Read the model definition and answer for the solid it produces. Units are mm, in the model's axes. A direction names the side the tool comes from. Round coordinates to 2 decimals unless told otherwise and drop trailing zeros. Order: outer loops, then holes, each group sorted by start corner. A loop starts at its lowest first (then second) coordinate and runs counter-clockwise, first axis right, second up. Notation, with made-up numbers: (-25, 89) -> (-5, 89) arc R11 cw to (-5, 101) -> close; hole circle Ø5 at (8, -18.75). An arc over 180 degrees is marked (long way). Use a Markdown table: item, result. Add a question column.
1. Section C-C, the plane z = 9.5 is taken. Give the vertices of the cut face in (x, y), then the cut area to 3 significant figures.
2. The mould has two halves that part along X. Classify faces 3 (the face through (-400, -200, -75)), 4 (the face through (419.524, -98.6, 70.664)), 5 (the face through (-419.524, -98.6, 79.336)): +X half, -X half, draft (parallel to the pull), parting line (faces both ways), or undercut.
3. Consider L1, parallel to Y at x = -26, z = 75.5; L2, parallel to X at y = -182, z = -71; L3, parallel to X at y = -56, z = 78.5. Determine where each line is inside the solid, lowest interval first. Write a range as [from, to].
4. Given pin 1 (3 mm diameter, centred on y = 56.5, z = 21, fed in from -X); pin 2 (8 mm diameter, centred on x = -234, z = -12, fed in from -Y), each flat-ended and moving along its own axis, determine where each tip first touches the part or whether it passes through.
5. Section D-D, the plane z = 75 is taken. Give the vertices of the cut face in (x, y), then the cut area to 3 significant figures.
6. Section A-A, the plane y = -19.5 is taken. Give the vertices of the cut face in (x, z), then the cut area to 3 significant figures.
7. Section B-B, the plane x = 400 is taken. Give the vertices of the cut face in (y, z).
8. For faces 1 (the face through (-380.476, -98.6, -79.336)), 2 (the face through (-7, 49, -125)), determine the directions among +Z, -Z, +X, -X, +Y, -Y from which every point of the face is accessible in a straight line to the end or side of a thin tool.
```python
from build123d import *

# Parameters (mm, degrees)
SKETCH1_W           = 1000
SKETCH1_H           = 250
BOSS_EXTRUDE1_DEPTH = 100
CUT_EXTRUDE1_DEPTH  = 568.89083458
SKETCH3_R           = 20
BOSS_EXTRUDE2_DEPTH = 200


with BuildPart() as part:
    # Sketch1 → Boss-Extrude1 (new body)
    with BuildSketch(Plane(origin=(0, 0, 0), x_dir=(1, 0, 0), z_dir=(0, 1, 0))):
        Rectangle(SKETCH1_W, SKETCH1_H)
    extrude(amount=BOSS_EXTRUDE1_DEPTH)

    # Sketch2 → Cut-Extrude1 (cut, through all)
    with BuildSketch(Plane.XY.offset(125)):
        with BuildLine():
            ThreePointArc((-500, 50), (-485.355339059, 85.355339059), (-450, 100))
            Line((-450, 100), (-500, 100))
            Line((-500, 100), (-500, 50))
        make_face()
        with BuildLine():
            ThreePointArc((-450, 0), (-485.355339059, 14.644660941), (-500, 50))
            Line((-500, 50), (-500, 0))
            Line((-500, 0), (-450, 0))
        make_face()
        with BuildLine():
            Line((500, 100), (450, 100))
            ThreePointArc((450, 100), (485.355339059, 85.355339059), (500, 50))
            Line((500, 50), (500, 100))
        make_face()
        with BuildLine():
            Line((500, 0), (500, 50))
            ThreePointArc((500, 50), (485.355339059, 14.644660941), (450, 0))
            Line((450, 0), (500, 0))
        make_face()
    extrude(amount=-CUT_EXTRUDE1_DEPTH, mode=Mode.SUBTRACT)

    # Sketch3 → Boss-Extrude2 (add)
    with BuildSketch(Plane.XZ):
        with Locations(Location((-400, 75, 0), (0, 0, 270))):
            Circle(SKETCH3_R)
        with Locations(Location((400, 75, 0), (0, 0, 90))):
            Circle(SKETCH3_R)
        with Locations(Location((400, -75, 0), (0, 0, 270))):
            Circle(SKETCH3_R)
        with Locations(Location((-400, -75, 0), (0, 0, 90))):
            Circle(SKETCH3_R)
    extrude(amount=BOSS_EXTRUDE2_DEPTH)


solid = part.part
```
Verdict:
| question | item | result |
|---|---|---|
| 1 | outline | (-450, 0) -> (450, 0) arc R50 ccw to (450, 100) -> (-450, 100) arc R50 ccw to start |
| 1 | area | 97,900 mm2 |
| 2 | face 3 | draft |
| 2 | face 4 | undercut |
| 2 | face 5 | undercut |
| 3 | L1 | y = [0, 100] |
| 3 | L2 | x = [-419.6, -380.4], [380.4, 419.6] |
| 3 | L3 | x = [-419.69, -380.31], [380.31, 419.69] |
| 4 | pin 1 | stops at x = -499.75 |
| 4 | pin 2 | stops at y = 0 |
| 5 | outline | (-450, 0) -> (-420, 0) -> (-420, -200) -> (-380, -200) -> (-380, 0) -> (380, 0) -> (380, -200) -> (420, -200) -> (420, 0) -> (450, 0) arc R50 ccw to (450, 100) -> (-450, 100) arc R50 ccw to start |
| 5 | area | 114,000 mm2 |
| 6 | outline | circle Ø40 at (-400, -75); circle Ø40 at (-400, 75); circle Ø40 at (400, -75); circle Ø40 at (400, 75) |
| 6 | area | 5,030 mm2 |
| 7 | outline | (-200, -95) -> (0, -95) -> (0, -125) -> (100, -125) -> (100, 125) -> (0, 125) -> (0, 95) -> (-200, 95) -> (-200, 55) -> (0, 55) -> (0, -55) -> (-200, -55) -> close |
| 8 | face 1 | -Y |
| 8 | face 2 | -Z, +X, -X, +Y, -Y |
